from build123d import *

# Parameters (mm, degrees)
SKETCH1_W           = 10
SKETCH1_H           = 12
SKETCH1_R           = 1.1
BOSS_EXTRUDE1_DEPTH = 4
FILLET1_R           = 2
SKETCH2_W           = 4
SKETCH2_H           = 12
BOSS_EXTRUDE2_DEPTH = 40


with BuildPart() as part:
    # Sketch1 → Boss-Extrude1 (new body)
    with BuildSketch(Plane.XY):
        Rectangle(SKETCH1_W, SKETCH1_H)
        Circle(SKETCH1_R, mode=Mode.SUBTRACT)
    extrude(amount=BOSS_EXTRUDE1_DEPTH)

    # Fillet1
    fillet1_edges = [part.edges().sort_by_distance(p)[0] for p in [
        (-5, 0, 4),
        (-5, 0, 0),
    ]]
    fillet(fillet1_edges, radius=FILLET1_R - 0.0001)  # a hair under: the kernel refuses the full size

    # Sketch2 → Boss-Extrude2 (add)
    with BuildSketch(Plane(origin=(5, 0, 0), x_dir=(0, 0, -1), z_dir=(1, 0, 0))):
        with Locations((-2, 0)):
            Rectangle(SKETCH2_W, SKETCH2_H)
    extrude(amount=BOSS_EXTRUDE2_DEPTH)


solid = part.part
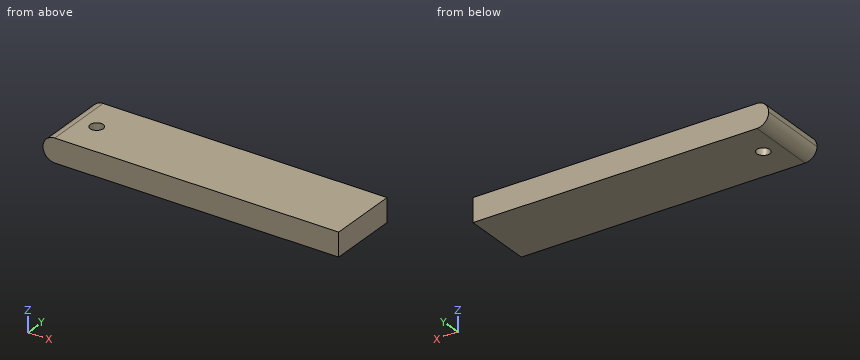
Can you work these out from the model? Positions are in its coordinate system, mm. Coordinates: 2 decimals unless noted, no trailing zeros. Write each loop counter-clockwise with the first axis right and the second up, starting at its lowest first coordinate (ties: lowest second). Pieces come first, ordered by that corner, then holes. Notation, with made-up numbers: (47, 29.5) - (89, 29.5) arc R13 cw to (89, 41.5) - close; hole circle Ø6 at (-34, 79). An arc over 180 degrees is marked (long way). Return JSON: item names as keys, results as strings. Group by question number.
Item 1: I'm going to push a flat-ended pin straight in: pin 1 Ø2 at (y, z) = (0.5, 3.5) entering from -X. Where does the tip first touch, or does it pass through?
Item 2: If we section it at B-B (x = 0): Write out the boundary of the cut face in (y, z).
Item 3: Please list where these lines run through material, in increasing order: probe 1 along Y at (x, z) = (0, 3.05); probe 2 along X at (y, z) = (-0.5, 2.1); probe 3 along X at (y, z) = (-0.25, 3.7).
Return value:
{
 "1": {"pin 1": "stops at x = -4.94"},
 "2": {"outline": "(-6, 0) - (-1.1, 0) - (-1.1, 4) - (-6, 4) - close; (1.1, 0) - (6, 0) - (6, 4) - (1.1, 4) - close"},
 "3": {"probe 1": "y = -6 to -1.1, 1.1 to 6", "probe 2": "x = -5 to -0.98, 0.98 to 45", "probe 3": "x = -4.05 to -1.07, 1.07 to 45"}
}
